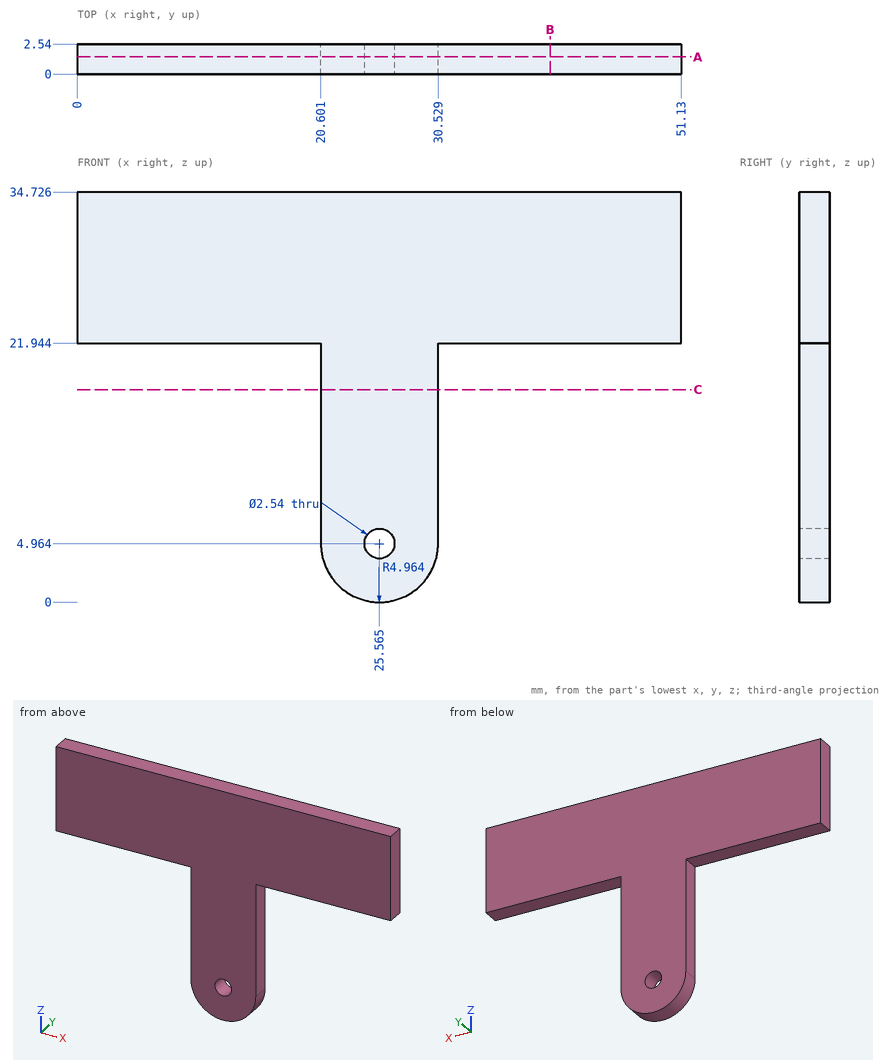
Geometry check sheet. Reference: drawing and pictorial views, mm from the part's lowest x, y, z. Round coordinates to 2 decimals unless told otherwise and drop trailing zeros. Loops run counter-clockwise (first coordinate to the right, second up) from the corner with the lowest first, then second, coordinate; pieces in that order, holes last. Notation, with made-up numbers: (-26, 71) - (22, 71) arc R13 cw to (22, 87) - close; hole circle Ø3 at (-27.5, 7.5). An arc over 180 degrees is marked (long way). Answer as CSV lines item,"result".
(1) Depth check by flat-ended pin: pin 1 Ø0.8 at (y, z) = (1.5, 14) entering from +X; pin 2 Ø1.5 at (y, z) = (2, 7) entering from -X; pin 3 Ø0.8 at (x, y) = (44.5, 1) entering from -Z. Enter the tip coordinate at first touch or a pass-through.
Output values:
pin 1,"stops at x = 30.53"
pin 2,"stops at x = 20.6"
pin 3,"stops at z = 21.94"
(2) Cross-section at A-A, the plane y = 1.45. Enter the section's corners in (x, z) (1 decimal), and give its area (3 significant figures).
Output values:
outline,"(0, 21.9) - (20.6, 21.9) - (20.6, 5) arc R5 ccw to (30.5, 5) - (30.5, 21.9) - (51.1, 21.9) - (51.1, 34.7) - (0, 34.7) - close; hole circle Ø2.5 at (25.6, 5)"
area,"856 mm²"
(3) Cross-section at C-C, the plane z = 18. Enter the section's corners in (x, y), and give its area (3 significant figures).
Output values:
outline,"(20.6, 0) - (30.53, 0) - (30.53, 2.54) - (20.6, 2.54) - close"
area,"25.2 mm²"
(4) Cross-section at B-B, the plane x = 40. Enter the section's corners in (y, z).
Output values:
outline,"(0, 21.94) - (2.54, 21.94) - (2.54, 34.73) - (0, 34.73) - close"
(5) Material ranges on line 1 along Z through (x, y) = (8, 0.8); line 2 along X through (y, z) = (0.6, 19); line 3 along X through (y, z) = (1.3, 4.5), recorded low to high.
Output values:
line 1,"z = 21.94 to 34.73"
line 2,"x = 20.6 to 30.53"
line 3,"x = 20.62 to 24.38, 26.75 to 30.51"
